```python
from build123d import *

# Parameters (mm, degrees)
SKETCH1_R                  = 50.8
BOSS_EXTRUDE1_DEPTH        = 3.175
F_6_0_204_DIAMETER_HOLE1_D = 5.1816
CIRPATTERN1_COUNT          = 6


with BuildPart() as part:
    # Sketch1 → Boss-Extrude1 (new body)
    with BuildSketch(Plane(origin=(0, 0, 0), x_dir=(1, 0, 0), z_dir=(0, 1, 0))):
        Circle(SKETCH1_R)
    extrude(amount=BOSS_EXTRUDE1_DEPTH)

    # #6 (0.204) Diameter Hole1 (through all)
    with Locations(Plane(origin=(0, 3.175, 0), x_dir=(1, 0, 0), z_dir=(0, 1, 0))):
        with Locations((0, 45.119902577)):
            f_6_0_204_diameter_hole1 = Hole(F_6_0_204_DIAMETER_HOLE1_D / 2)

    # CirPattern1: #6 (0.204) Diameter Hole1 ×6 about axis
    cirpattern1_axis = Axis((0, 0, 0), (0, 1, 0))
    for i in range(1, CIRPATTERN1_COUNT):
        add(f_6_0_204_diameter_hole1.rotate(cirpattern1_axis, i * 360 / CIRPATTERN1_COUNT), mode=Mode.SUBTRACT)


solid = part.part
```
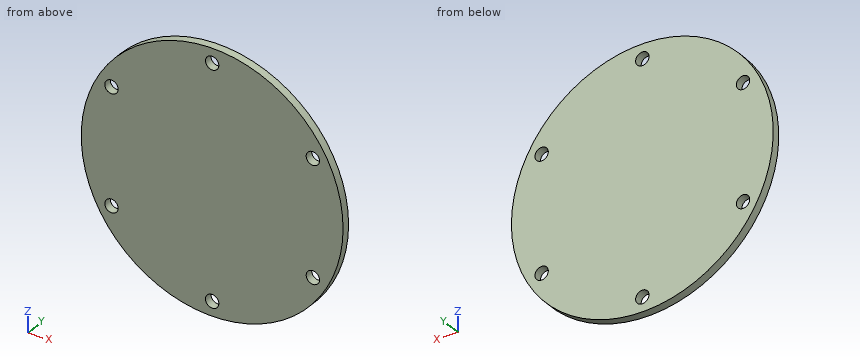
Verification items for the finished model (mm, model axes). Round coordinates to 2 decimals unless told otherwise and drop trailing zeros. Write each loop counter-clockwise with the first axis right and the second up, starting at its lowest first coordinate (ties: lowest second). Pieces come first, ordered by that corner, then holes. Notation, with made-up numbers: (47, 19.25) -> (75, 19.25) arc R10 ccw to (75, 24.25) -> close; hole circle Ø9 at (38.5, 86). An arc over 180 degrees is marked (long way). Write each question's results on one line, items separated by ' | '. Start each with the question number.
1. Cross-section at C-C (z = -11.5). Enter the section's corners in (x, y) (3 decimals).
2. Material ranges on probe 1 along Z at (x, y) = (0, 2.15); probe 2 along Z at (x, y) = (-1.5, 0.75); probe 3 along X at (y, z) = (1.15, -43.5), recorded low to high. Write a range as from..to.
3. Depth check by flat-ended pin: P1, Ø4, axis at x = -39.07, z = 22.56, coming from the +Y side; P2, Ø1, axis at x = 22.5, y = 2.5, coming from the -Z side; P3, Ø1, axis at y = 0.5, z = 31.5, coming from the +X side; P4, Ø1, axis at x = -21.5, y = 2, coming from the +Z side. Enter the tip coordinate at first touch or a pass-through.
4. Cross-section at A-A (x = 0). Enter the section's corners in (y, z) (3 decimals).
5. Cross-section at B-B (y = 2). Enter the section's corners in (x, z), then the cut area to 3 significant figures.
6. Cross-section at D-D (x = -11). Enter the section's corners in (y, z) (3 decimals), then the cut area to 3 significant figures.
Solutions:
1) outline: (-49.481, 0) -> (49.481, 0) -> (49.481, 3.175) -> (-49.481, 3.175) -> close
2) probe 1: z = -50.8..-47.71, -42.53..42.53, 47.71..50.8 | probe 2: z = -50.78..-47.23, -43.01..43.01, 47.23..50.78 | probe 3: x = -26.24..-2.02, 2.02..26.24
3) P1: passes through | P2: stops at z = -45.79 | P3: stops at x = 40.24 | P4: stops at z = 46.26
4) outline: (0, -50.8) -> (3.175, -50.8) -> (3.175, -47.711) -> (0, -47.711) -> close; (0, -42.529) -> (3.175, -42.529) -> (3.175, 42.529) -> (0, 42.529) -> close; (0, 47.711) -> (3.175, 47.711) -> (3.175, 50.8) -> (0, 50.8) -> close
5) outline: circle Ø101.6 at (0, 0); hole circle Ø5.18 at (-39.07, -22.56); hole circle Ø5.18 at (-39.07, 22.56); hole circle Ø5.18 at (0, -45.12); hole circle Ø5.18 at (0, 45.12); hole circle Ø5.18 at (39.07, -22.56); hole circle Ø5.18 at (39.07, 22.56) | area: 7,980 mm2
6) outline: (0, -49.595) -> (3.175, -49.595) -> (3.175, 49.595) -> (0, 49.595) -> close | area: 315 mm2
